Check sheet for the modelled part. Datum: model origin and axes. Units: mm. Give positions to 0.01 mm unless a question says otherwise; leave off trailing zeros. Loops run counter-clockwise (first coordinate to the right, second up) from the corner with the lowest first, then second, coordinate; pieces in that order, holes last.
```python
from build123d import *

# Parameters (mm, degrees)
F1_R = 6.35
F3_T = -1.27


with BuildPart() as f2:
    # F2: sweep along a path in F0
    with BuildLine(Plane.XZ) as f2_path:
        Line((-23.1357552849, 0), (-23.1357552849, 2.54))
        ThreePointArc((-23.1357552849, 2.54), (0, 25.6757552849), (23.1357552849, 2.54))
        Line((23.1357552849, 2.54), (23.1357552849, 0))
    # F1 (on Top) → F2 (sweep)
    with BuildSketch(Plane.XY):
        with Locations((23.1357552849, 0)):
            Circle(F1_R)
    sweep(path=f2_path.line)

    # F3
    f3_openings = [f2.faces().sort_by_distance(p)[0] for p in [
        (-23.135755, 0, 0),
        (23.135755, 0, 0),
    ]]
    offset(amount=F3_T, openings=f3_openings)


solid = f2.part
```
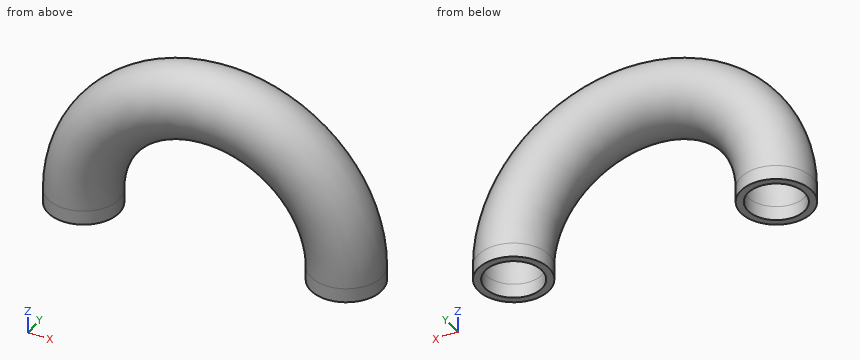
(1) Material ranges on line 1 (X direction, y = 2.25, z = 7); line 2 (X direction, y = -0.5, z = 11.5); line 3 (X direction, y = -4, z = 23), recorded low to high.
(2) Section check B-B on y = -3. Record the boundary of the cut face in (x, z), plus the area to 3 significant figures.
(3) Gauge pin test, flat ends, axial feed: pin 1 Ø1 at (x, z) = (-20.5, 23.5) entering from +Y; pin 2 Ø8 at (x, z) = (15, 15.5) entering from +Y; pin 3 Ø3 at (y, z) = (3, 21.5) entering from +X; pin 4 Ø1 at (y, z) = (2.5, 6) entering from +X. Record the tip position at first contact, or that the pin passes through.
(4) Section check C-C on z = 8.5. Give the number of separate pieces and of enclosed holes in the cut face, plus the area to 3 significant figures.
(5) Section check A-A on y = 0. Record the boundary of the cut face in (x, z).
Computed values:
1. line 1: x = -28.73 to -27.33, -18.04 to -16.61, 16.61 to 18.04, 27.33 to 28.73
1. line 2: x = -28.07 to -26.73, -15.7 to -14.22, 14.22 to 15.7, 26.73 to 28.07
1. line 3: x = -19.21 to -16.47, 16.47 to 19.21
2. outline: (-28.73, 0) - (-27.24, 0) - (-27.24, 2.54) arc R27.24 cw to (27.24, 2.54) - (27.24, 0) - (28.73, 0) - (28.73, 2.54) arc R28.73 ccw to (-28.73, 2.54) - close; (-19.04, 0) - (-17.54, 0) - (-17.54, 2.54) arc R17.54 cw to (17.54, 2.54) - (17.54, 0) - (19.04, 0) - (19.04, 2.54) arc R19.04 ccw to (-19.04, 2.54) - close
2. area: 233 mm2
3. pin 1: stops at y = 2.83
3. pin 2: stops at y = 6.35
3. pin 3: stops at x = 23.1
3. pin 4: stops at x = 28.97
4. separate pieces: 2
4. enclosed holes: 2
4. area: 94.8 mm2
5. outline: (-29.49, 0) - (-28.22, 0) - (-28.22, 2.54) arc R28.22 cw to (28.22, 2.54) - (28.22, 0) - (29.49, 0) - (29.49, 2.54) arc R29.49 ccw to (-29.49, 2.54) - close; (-18.06, 0) - (-16.79, 0) - (-16.79, 2.54) arc R16.79 cw to (16.79, 2.54) - (16.79, 0) - (18.06, 0) - (18.06, 2.54) arc R18.06 ccw to (-18.06, 2.54) - close
